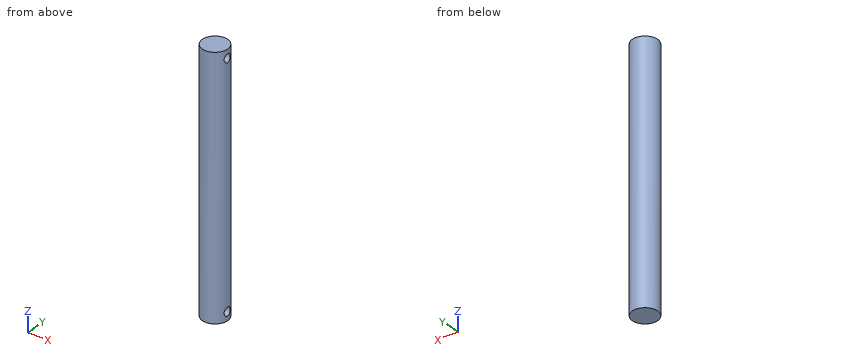
Solid Edge part; units mm, degrees
sketch "Sketch1" plane through (0, 0, 0) normal (0, 0, 1) x (1, 0, 0)
  circle A0 centre (0, 0) radius 7.5
extrude "Protrusion1" add sketch "Sketch1" along normal blind 150
hole "Hole_4" at (0, 0, 145) direction (1, 0, 0) diameter 4.917 depth 7.5
hole "Hole1" at (0, 0, 5) direction (1, 0, 0) diameter 4.917 depth 7.5
Here's how the part is built. I have some questions about the finished solid (model axes, mm). Give positions to 0.01 mm unless a question says otherwise; leave off trailing zeros. Order: outer loops, then holes, each group sorted by start corner. A loop starts at its lowest first (then second) coordinate and runs counter-clockwise, first axis right, second up. Notation, with made-up numbers: (-20.75, 52.5) -> (-8.75, 52.5) arc R22 cw to (-8.75, 91.5) -> close; hole circle Ø8 at (71, 17.5). An arc over 180 degrees is marked (long way). One line per item, written item: value. Start each with the question number.
1. Imagine slicing it at B-B, the plane z = 130.5. List the corners of the cut face in (x, y) for me.
2. Imagine slicing it at A-A, the plane x = 4.75. List the corners of the cut face in (y, z) for me, plus the area to 3 significant figures.
3. Imagine slicing it at C-C, the plane x = -4.5. List the corners of the cut face in (y, z) for me, plus the area to 3 significant figures.
4. I need wall thicknesses on probe 1 along Z at (x, y) = (2, 0); probe 2 along X at (y, z) = (-0.25, 127); probe 3 along Z at (x, y) = (5.75, -1.5). Which ranges of each line are inside material? Lowest first, please. Write a range as from..to.
5. Will these pins go through, and if not, where does the flat tip stop? pin 1 Ø1.5 at (x, z) = (1.5, 16.5) entering from +Y; pin 2 Ø5 at (y, z) = (-4.5, 122.5) entering from +X; pin 3 Ø2 at (x, z) = (-2.5, 65.5) entering from +Y.
6. Imagine slicing it at D-D, the plane y = -4. List the corners of the cut face in (x, z) for me.
Values follow:
1. outline: circle Ø15 at (0, 0)
2. outline: (-5.8, 0) -> (5.8, 0) -> (5.8, 150) -> (-5.8, 150) -> close; hole circle Ø4.92 at (0, 5); hole circle Ø4.92 at (0, 145)
2. area: 1,700 mm2
3. outline: (-6, 0) -> (6, 0) -> (6, 150) -> (-6, 150) -> close
3. area: 1,800 mm2
4. probe 1: z = 0..2.54, 7.46..142.54, 147.46..150
4. probe 2: x = -7.5..7.5
4. probe 3: z = 0..3.05, 6.95..143.05, 146.95..150
5. pin 1: stops at y = 7.46
5. pin 2: stops at x = 7.23
5. pin 3: stops at y = 7.35
6. outline: (-6.34, 0) -> (6.34, 0) -> (6.34, 150) -> (-6.34, 150) -> close
